Geometry check sheet. Reference: drawing and pictorial views, mm from the part's lowest x, y, z. A direction names the side the tool comes from. Round coordinates to 2 decimals unless told otherwise and drop trailing zeros. Write each loop counter-clockwise with the first axis right and the second up, starting at its lowest first coordinate (ties: lowest second). Pieces come first, ordered by that corner, then holes. Notation, with made-up numbers: M 69.5,-5 L 101.5,-5 A34 cw 101.5,29 Z; hole C -14,79 d5. An arc over 180 degrees is marked long. Answer in a Markdown table with one row per item.
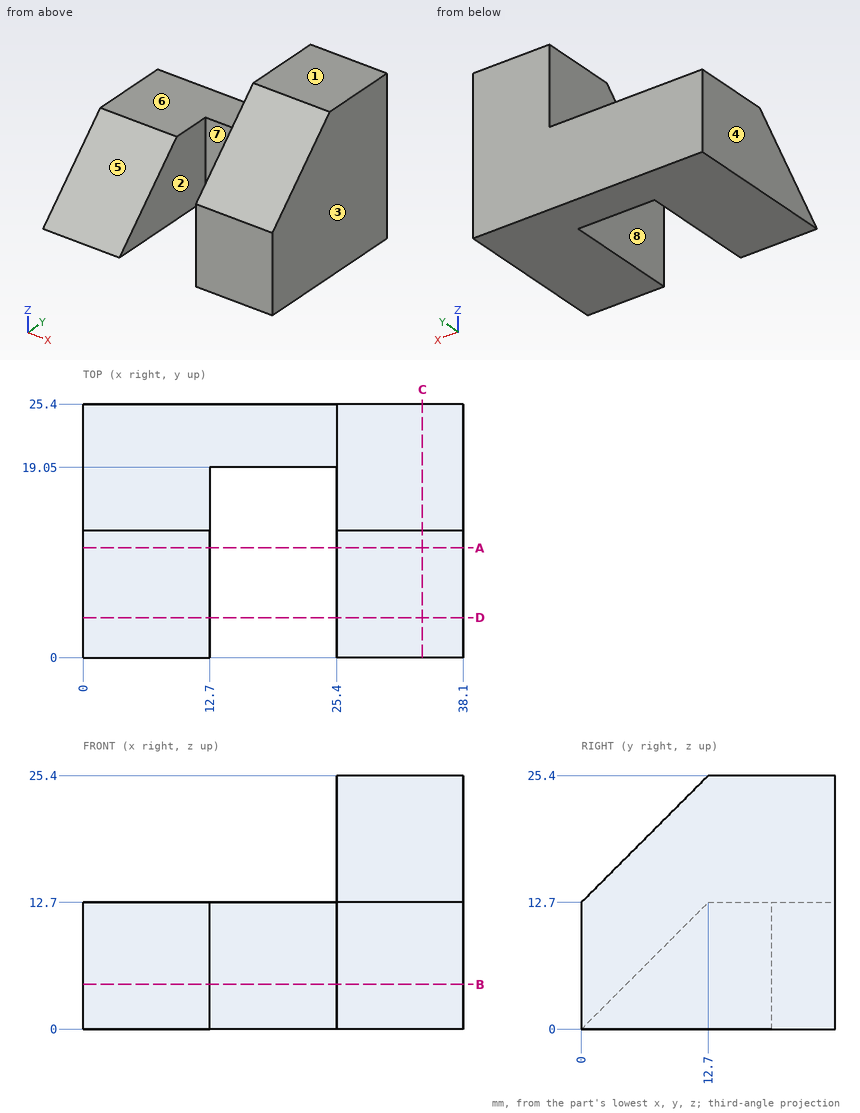
1. Section check C-C, the plane x = 34. Record the cut outline in (y, z), and give its area (3 significant figures).
Found:
| item | result |
|---|---|
| outline | M 0,0 L 25.4,0 L 25.4,25.4 L 12.7,25.4 L 0,12.7 Z |
| area | 565 mm2 |
2. Section check D-D, the plane y = 4. Record the cut outline in (x, z).
Found:
| item | result |
|---|---|
| outline | M 0,0 L 12.7,0 L 12.7,4 L 0,4 Z; M 25.4,0 L 38.1,0 L 38.1,16.7 L 25.4,16.7 Z |
3. Scan lines: L1, parallel to Z at x = 9, y = 15.5; L2, parallel to X at y = 13.25, z = 23; L3, parallel to X at y = 10.75, z = 6. Record each from-to range of solid material in increasing order.
Found:
| item | result |
|---|---|
| L1 | z = 0 to 12.7 |
| L2 | x = 25.4 to 38.1 |
| L3 | x = 0 to 12.7, 25.4 to 38.1 |
4. Section check B-B, the plane z = 4.5. Record the cut outline in (x, y).
Found:
| item | result |
|---|---|
| outline | M 0,4.5 L 12.7,4.5 L 12.7,19.05 L 25.4,19.05 L 25.4,0 L 38.1,0 L 38.1,25.4 L 0,25.4 Z |
5. Go/stop test with flat-tipped pins: pin 1 (4 mm diameter, centred on x = 19.5, z = 7, fed in from -Y); pin 2 (5 mm diameter, centred on x = 9.5, y = 11, fed in from +Z). Record where each tip stops, or that it passes through.
Found:
| item | result |
|---|---|
| pin 1 | stops at y = 19.05 |
| pin 2 | stops at z = 12.7 |
6. Section check A-A, the plane y = 11. Record the cut outline in (x, z).
Found:
| item | result |
|---|---|
| outline | M 0,0 L 12.7,0 L 12.7,11 L 0,11 Z; M 25.4,0 L 38.1,0 L 38.1,23.7 L 25.4,23.7 Z |
7. Access from +Z, -Z, +X, -X, +Y, -Y to the whole of each face (thin tool, end or side, straight path). Record for the marked faces 5, 6, 7 and 8.
Found:
| item | result |
|---|---|
| face 5 | +Z, -X, -Y |
| face 6 | +Z, -X, +Y, -Y |
| face 7 | +Z, -Z, -Y |
| face 8 | +Z, -Y |
8. Draft check along X on the marked faces 1, 2, 3 and 4. Enter one of: +X half, -X half, draft (parallel to the pull), parting line (faces both ways), or undercut.
Found:
| item | result |
|---|---|
| face 1 | draft |
| face 2 | undercut |
| face 3 | +X half |
| face 4 | -X half |
